Part model, mm, in its own coordinate system. A direction names the side the tool comes from. Give positions to 0.01 mm unless a question says otherwise; leave off trailing zeros. Write each loop counter-clockwise with the first axis right and the second up, starting at its lowest first coordinate (ties: lowest second). Pieces come first, ordered by that corner, then holes. Notation, with made-up numbers: (81.5, -1) - (110.5, -1) arc R21 ccw to (110.5, 8) - close; hole circle Ø5 at (33, 1.5). An arc over 180 degrees is marked (long way). Answer in a Markdown table with one row per item. Add a question column.
1. Band-saw the part on B-B on z = 229.5. Write the cut outline in (x, y), plus the area to 3 significant figures.
2. Probe line 1 along X through (y, z) = (-2.25, 137.5); line 2 along Y through (x, z) = (-4.75, 105); line 3 along Y through (x, z) = (5.5, 13.5). List the from-to ranges inside material, lowest first.
3. Drop flat-ended pins along their axis: pin 1 Ø1.8 at (x, z) = (0, 237.5) entering from +Y; pin 2 Ø4 at (x, z) = (0, 187.5) entering from +Y. Give the stop position or say it passes through.
4. Which spindle directions (+Z, -Z, +X, -X, +Y, -Y) get a long thin tool onto all of the face, cutting with end or side? Do faces 5 (the flat face through (-6, -2, 123)), 6 (the flat face through (2, -0.5, 137)). Say none if no direction does.
5. Pull direction Z, two halves, no side cores. Call faces 1 (the flat face through (2, -0.5, 62)), 2 (the flat face through (0, 0, 0)), 3 (the cylindrical face through (-0.391, 1.781, 34.526)), 4 (the flat face through (6, -2, 123)): released by +Z, released by -Z, zero draft, split by the parting line, or undercut.
6. Band-saw the part on A-A on y = -1.75. State how many separate pieces and enclosed holes the cut face has, plus the area to 3 significant figures.
```python
from build123d import *

# Parameters (mm, degrees)
EXTRUDE_1_DEPTH        = 250
SKETCH_2_R             = 3
SKETCH_2_R_2           = 1.75
CUT_EXTRUDE_1_DEPTH    = 4.5
SKETCH_2_2_R           = 1.75
CUT_EXTRUDE_2_DEPTH    = 9
PATTERN_LINEAR_1_COUNT = 10
PATTERN_LINEAR_1_PITCH = 25


with BuildPart() as part:
    # Эскиз1 → Бобышка-Вытянуть1 (new body)
    with BuildSketch(Plane.XY):
        with BuildLine():
            Line((-6, 3.7), (-5.7, 4))
            Line((-5.7, 4), (5.7, 4))
            Line((5.7, 4), (6, 3.7))
            Line((6, 3.7), (6, 2.451013544))
            ThreePointArc((6, 2.451013544), (5.597935912, 2.202976267), (5.354599002, 1.798050138))
            Line((5.354599002, 1.798050138), (4.643514056, 1.798050138))
            Line((4.643514056, 1.798050138), (4.643514056, 1.201949862))
            Line((4.643514056, 1.201949862), (5.354599002, 1.201949862))
            ThreePointArc((5.354599002, 1.201949862), (5.597935912, 0.797023733), (6, 0.548986456))
            Line((6, 0.548986456), (6, -3.7))
            Line((6, -3.7), (5.7, -4))
            Line((5.7, -4), (-5.7, -4))
            Line((-5.7, -4), (-6, -3.7))
            Line((-6, -3.7), (-6, 0.548986456))
            ThreePointArc((-6, 0.548986456), (-5.597935912, 0.797023733), (-5.354599002, 1.201949862))
            Line((-5.354599002, 1.201949862), (-4.643514056, 1.201949862))
            Line((-4.643514056, 1.201949862), (-4.643514056, 1.798050138))
            Line((-4.643514056, 1.798050138), (-5.354599002, 1.798050138))
            ThreePointArc((-5.354599002, 1.798050138), (-5.597935912, 2.202976267), (-6, 2.451013544))
            Line((-6, 2.451013544), (-6, 3.7))
        make_face()
    extrude(amount=EXTRUDE_1_DEPTH)

    # Эскиз2 → Вырез-Вытянуть1 (cut)
    with BuildSketch(Plane(origin=(0, 4, 0), x_dir=(1, 0, 0), z_dir=(0, 1, 0))):
        with Locations((0, -12.5)):
            Circle(SKETCH_2_R)
        with Locations((0, -12.5)):
            Circle(SKETCH_2_R_2, mode=Mode.SUBTRACT)
    cut_extrude_1 = extrude(amount=-CUT_EXTRUDE_1_DEPTH, mode=Mode.SUBTRACT)

    # Эскиз2<2> → Вырез-Вытянуть2 (cut, through all)
    with BuildSketch(Plane(origin=(0, 4, 0), x_dir=(1, 0, 0), z_dir=(0, 1, 0))):
        with Locations((0, -12.5)):
            Circle(SKETCH_2_2_R)
    cut_extrude_2 = extrude(amount=-CUT_EXTRUDE_2_DEPTH, mode=Mode.SUBTRACT)

    # Линейный массив1: Вырез-Вытянуть1, Вырез-Вытянуть2 ×10
    with Locations(*[(0, 0, i * PATTERN_LINEAR_1_PITCH) for i in range(1, PATTERN_LINEAR_1_COUNT)]):
        add(cut_extrude_1, mode=Mode.SUBTRACT)
        add(cut_extrude_2, mode=Mode.SUBTRACT)


solid = part.part
```
Values:
| question | item | result |
|---|---|---|
| 1 | outline | (-6, -3.7) - (-5.7, -4) - (5.7, -4) - (6, -3.7) - (6, 0.55) arc R1 cw to (5.35, 1.2) - (4.64, 1.2) - (4.64, 1.8) - (5.35, 1.8) arc R1 cw to (6, 2.45) - (6, 3.7) - (5.7, 4) - (-5.7, 4) - (-6, 3.7) - (-6, 2.45) arc R1 cw to (-5.35, 1.8) - (-4.64, 1.8) - (-4.64, 1.2) - (-5.35, 1.2) arc R1 cw to (-6, 0.55) - close |
| 1 | area | 93.1 mm² |
| 2 | line 1 | x = -6 to -1.75, 1.75 to 6 |
| 2 | line 2 | y = -4 to 1.2, 1.8 to 4 |
| 2 | line 3 | y = -4 to 0.91, 2.09 to 4 |
| 3 | pin 1 | passes through |
| 3 | pin 2 | stops at y = -0.5 |
| 4 | face 5 | +Z, -Z, -X, +Y, -Y |
| 4 | face 6 | +Y |
| 5 | face 1 | undercut |
| 5 | face 2 | released by -Z |
| 5 | face 3 | undercut |
| 5 | face 4 | zero draft |
| 6 | separate pieces | 1 |
| 6 | enclosed holes | 10 |
| 6 | area | 2,900 mm² |
